Can you work these out from the model? Positions are in its coordinate system, mm. A direction names the side the tool comes from. Coordinates: 2 decimals unless noted, no trailing zeros. Loops run counter-clockwise (first coordinate to the right, second up) from the corner with the lowest first, then second, coordinate; pieces in that order, holes last. Notation, with made-up numbers: M -18.5,4 L 33.5,4 A14 ccw 33.5,25 Z; hole C 2.25,-10 d8. An arc over 180 degrees is marked long. Answer as a JSON object with one key per item and string values. Group by question number.
Item 1: Which directions (+Z, -Z, +X, -X, +Y, -Y) give clear straight access to the entire face, cutting with the end or side of a thin tool? Please do faces 4 (the flat face through (8, 21, 7.938)), 5 (the flat face through (13.918, 1.957, 3.913)), 6 (the cylindrical face through (2.387, 64.412, 4.08)), 7 (the flat face through (8, -3.969, 4)), 8 (the flat face through (2, -11, 4.813)).
Item 2: If I drill on line 1 (X direction, y = -4, z = 5.25) (3 decimals); line 2 (Y direction, x = 13, z = 2); line 3 (Y direction, x = 2.5, z = 2), over which ranges is the centre line in solid material (lowest first)?
Item 3: Suppose I cut it at D-D (x = 5). Write out the boundary of the cut face in (y, z).
Item 4: Suppose I cut it at B-B (x = 14.75). Write out the boundary of the cut face in (y, z) (1 decimal), then the cut area to 3 significant figures.
Item 5: Suppose I cut it at A-A (y = -6). Write out the boundary of the cut face in (x, z) (1 decimal), then the cut area to 3 significant figures.
Item 6: We'd pull the mould along Z, two halves only. Please class faces 1 (the flat face through (8, 59, 11.906)), 2 (the flat face through (2, -10, 1.556)), 3 (the flat face through (15.875, -5, 4)): +Z half, -Z half, draft (parallel to the pull), parting line (faces both ways), or undercut.
Item 7: I'm going to push flat-ended pins straight in: pin 1 Ø1.5 at (x, y) = (5, 17) entering from -Z; pin 2 Ø3 at (y, z) = (12, 0) entering from +X; pin 3 Ø8 at (x, z) = (12.5, 8) entering from +Y. Where does each tip first touch, or does it pass through?
```python
from build123d import *

# Parameters (mm, degrees)
F1_DEPTH = 7.9375
F2_R     = 2.54
F2_W     = 1.6891
F2_H     = 1.56845
F2_H_2   = 1.6891
F2_W_2   = 1.56845
F3_DEPTH = 15.875
F4_SIZE  = 3.96874
F5_W     = 15.875
F5_H     = 15.875
F6_DEPTH = 15.875
F7_R     = 7.93749


# Not quite as in the source:
# - a fillet or chamfer is up to 0.001 mm smaller than in the source, because OpenCascade refuses the exact size


with BuildPart() as f1:
    # F0 (on Top) → F1 (new body)
    with BuildSketch(Plane.XY):
        Polygon((3.96875, 0), (0, 0), (0, -13.49375), (3.96875, -13.49375), (3.96875, -3.96875), (11.90625, -3.96875), (11.90625, -13.49375), (15.875, -13.49375), (15.875, 0), (11.90625, 0), (11.90625, 50.8), (3.96875, 50.8), align=None)
    extrude(amount=F1_DEPTH)

    # F2 (on face) → F3 (cut, through all)
    with BuildSketch(Plane.YZ.offset(15.875)):
        with BuildLine():
            ThreePointArc((-9.525, 0), (-12.3313300378, 1.1624199622), (-13.49375, 3.96875))
            Line((-13.49375, 3.96875), (-13.49375, 0))
            Line((-13.49375, 0), (-9.525, 0))
        make_face()
        with BuildLine():
            ThreePointArc((-13.49375, 3.96875), (-12.3313300378, 6.7750800378), (-9.525, 7.9375))
            Line((-9.525, 7.9375), (-13.49375, 7.9375))
            Line((-13.49375, 7.9375), (-13.49375, 3.96875))
        make_face()
        with Locations((14.128559196, 3.96875)):
            Circle(F2_R)
        with Locations((-9.525, 5.597525)):
            Rectangle(F2_W, F2_H)
        with Locations((-9.525, 3.96875)):
            Rectangle(F2_W, F2_H_2)
        with Locations((-11.153775, 3.96875)):
            Rectangle(F2_W_2, F2_H_2)
        with Locations((-7.896225, 3.96875)):
            Rectangle(F2_W_2, F2_H_2)
        with Locations((-9.525, 2.339975)):
            Rectangle(F2_W, F2_H)
    extrude(amount=-F3_DEPTH, mode=Mode.SUBTRACT)

    # F4 (size 3.96875 in the source; OpenCascade refuses exactly that, so slightly less here)
    f4_edges = [f1.edges().sort_by_distance(p)[0] for p in [
        (11.90625, 0, 3.96875),
        (3.96875, 0, 3.96875),
    ]]
    chamfer(f4_edges, length=F4_SIZE)

    # F5 (on face) → F6 (join)
    with BuildSketch(Plane(origin=(0, 50.8, 0), x_dir=(-1, 0, 0), z_dir=(0, 1, 0))):
        with Locations((-7.9375, 3.96875)):
            Rectangle(F5_W, F5_H)
    extrude(amount=F6_DEPTH)

    # F7 (radius 7.9375 in the source; OpenCascade refuses exactly that, so slightly less here)
    f7_edges = [f1.edges().sort_by_distance(p)[0] for p in [
        (15.875, 66.675, 3.96875),
        (0, 66.675, 3.96875),
    ]]
    fillet(f7_edges, radius=F7_R)


solid = f1.part
```
From the geometry:
{
 "1": {"face 4": "+Z, +X, -X, -Y", "face 5": "+Z, -Z, +X", "face 6": "+Z, -Z, -X, +Y", "face 7": "+Z, -Z, -Y", "face 8": "+X, -X"},
 "2": {"line 1": "0 to 3.969, 11.906 to 15.875", "line 2": "-12.97 to -10.37, -8.68 to 2.87, 50.8 to 64.85", "line 3": "-12.97 to -10.37, -8.68 to 2.5, 50.8 to 64.52"},
 "3": {"outline": "M -3.97,0 L 50.8,0 L 50.8,-3.97 L 66.11,-3.97 L 66.11,11.91 L 50.8,11.91 L 50.8,7.94 L -3.97,7.94 Z; hole C 14.13,3.97 d5.08"},
 "4": {"outline": "M -9.5,0 L 1.1,0 L 1.1,7.9 L -9.5,7.9 A4 ccw Z; M 50.8,-4 L 62.8,-4 L 62.8,11.9 L 50.8,11.9 Z; hole M -11.9,3.1 L -10.4,3.1 L -10.4,1.6 L -8.7,1.6 L -8.7,3.1 L -7.1,3.1 L -7.1,4.8 L -8.7,4.8 L -8.7,6.4 L -10.4,6.4 L -10.4,4.8 L -11.9,4.8 Z", "area": "287 mm2"},
 "5": {"outline": "M 0,0 L 4,0 L 4,7.9 L 0,7.9 Z; M 11.9,0 L 15.9,0 L 15.9,7.9 L 11.9,7.9 Z", "area": "63.0 mm2"},
 "6": {"face 1": "+Z half", "face 2": "undercut", "face 3": "draft"},
 "7": {"pin 1": "z = 0", "pin 2": "x = 11.91", "pin 3": "y = 66.66"}
}
